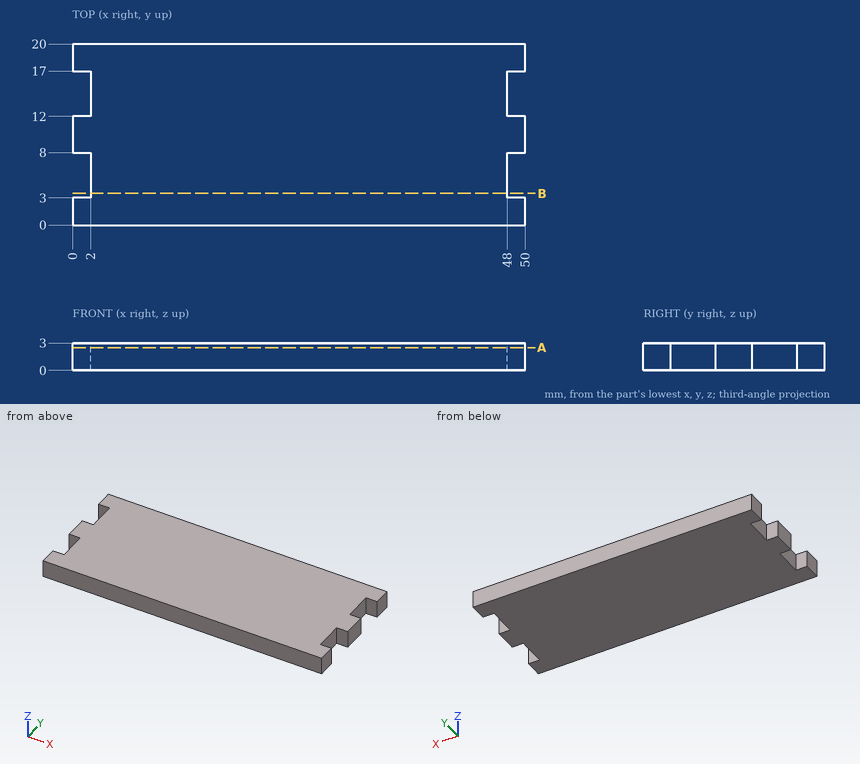
Design review of the part shown in the three views and the two pictorial views. Dimensions are in mm from the part's minimum x, y and z. Round coordinates to 2 decimals unless told otherwise and drop trailing zeros. Write each loop counter-clockwise with the first axis right and the second up, starting at its lowest first coordinate (ties: lowest second). Pieces come first, ordered by that corner, then holes.
1) Take a section at B-B on y = 3.5. Give the boundary of the cut face in (x, z), then the cut area to 3 significant figures.
Answer below:
outline: (2, 0) - (48, 0) - (48, 3) - (2, 3) - close
area: 138 mm2
2) For line 1 along Y through (x, z) = (48.5, 2.05); line 2 along X through (y, z) = (5.5, 0.75), list the stretches that pass through material, from the lowest coordinate up.
Answer below:
line 1: y = 0 to 3, 8 to 12, 17 to 20
line 2: x = 2 to 48
3) Take a section at A-A on z = 2.5. Give the boundary of the cut face in (x, y).
Answer below:
outline: (0, 0) - (50, 0) - (50, 3) - (48, 3) - (48, 8) - (50, 8) - (50, 12) - (48, 12) - (48, 17) - (50, 17) - (50, 20) - (0, 20) - (0, 17) - (2, 17) - (2, 12) - (0, 12) - (0, 8) - (2, 8) - (2, 3) - (0, 3) - close
